Verification items for this drawing (mm, ordinates from the low corner). A direction names the side the tool comes from. Round coordinates to 2 decimals unless told otherwise and drop trailing zeros. Order: outer loops, then holes, each group sorted by start corner. A loop starts at its lowest first (then second) coordinate and runs counter-clockwise, first axis right, second up. Notation, with made-up numbers: (-3.75, -4) - (41.25, -4) arc R22 cw to (41.25, 20) - close; hole circle Ø8 at (-3.5, -32.75). An arc over 180 degrees is marked (long way). Answer as CSV lines item,"result". Start each with the question number.
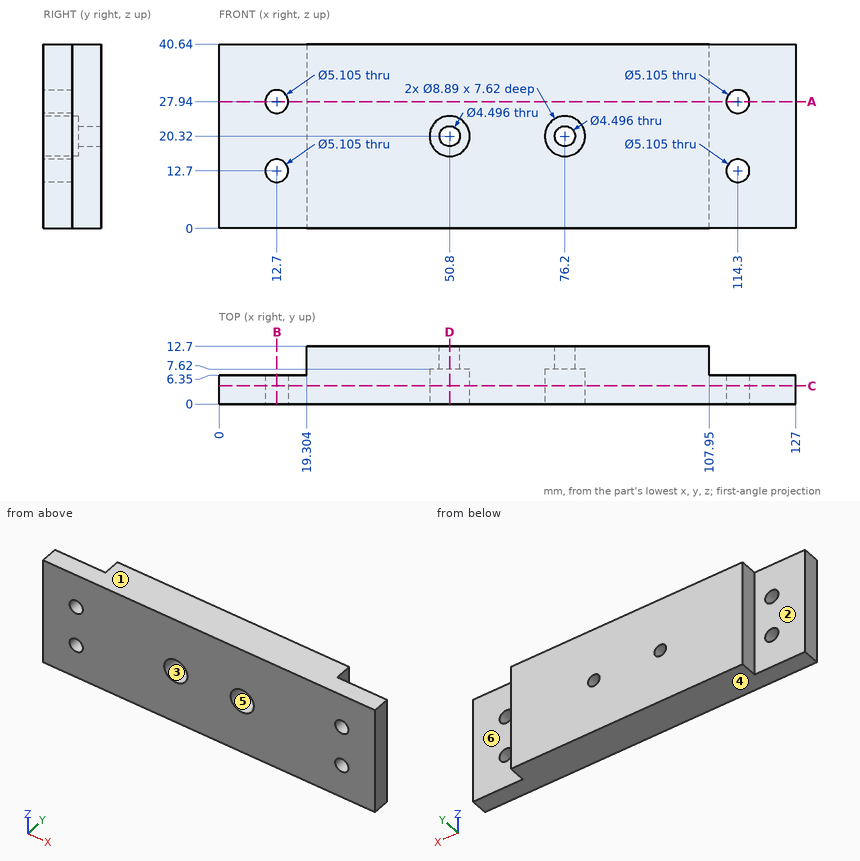
1. Section check B-B on x = 12.7. Record the boundary of the cut face in (y, z).
2. Section check D-D on x = 50.8. Record the boundary of the cut face in (y, z) (1 decimal).
3. Section check C-C on y = 4. Record the boundary of the cut face in (x, z) (1 decimal).
4. Go/stop test with flat-tipped pins: pin 1 Ø5 at (y, z) = (11, 20) entering from -X; pin 2 Ø8 at (x, z) = (114.3, 12.7) entering from +Y; pin 3 Ø2.5 at (x, z) = (50, 22.5) entering from -Y. Record where each tip stops, or that it passes through.
5. Thickness scan on probe 1 along X at (y, z) = (9.25, 20.32); probe 2 along Z at (x, y) = (50.8, 3.75) (1 decimal); probe 3 along X at (y, z) = (1.75, 27.94). Record the ranges inside material, lowest first.
6. Access from +Z, -Z, +X, -X, +Y, -Y to the whole of each face (thin tool, end or side, straight path). Record for the marked faces 1 and 2.
7. Section check A-A on z = 27.94. Record the boundary of the cut face in (x, y).
8. Draft check along Z on the marked faces 3, 4, 5 and 6. Enter one of: released by +Z, released by -Z, zero draft, split by the parting line, or undercut.
Numbers:
1,outline,"(0, 0) - (6.35, 0) - (6.35, 10.15) - (0, 10.15) - close; (0, 15.25) - (6.35, 15.25) - (6.35, 25.39) - (0, 25.39) - close; (0, 30.49) - (6.35, 30.49) - (6.35, 40.64) - (0, 40.64) - close"
2,outline,"(0, 0) - (12.7, 0) - (12.7, 18.1) - (7.6, 18.1) - (7.6, 15.9) - (0, 15.9) - close; (0, 24.8) - (7.6, 24.8) - (7.6, 22.6) - (12.7, 22.6) - (12.7, 40.6) - (0, 40.6) - close"
3,outline,"(0, 0) - (127, 0) - (127, 40.6) - (0, 40.6) - close; hole circle Ø5.1 at (12.7, 12.7); hole circle Ø5.1 at (12.7, 27.9); hole circle Ø8.9 at (50.8, 20.3); hole circle Ø8.9 at (76.2, 20.3); hole circle Ø5.1 at (114.3, 12.7); hole circle Ø5.1 at (114.3, 27.9)"
4,pin 1,"stops at x = 19.3"
4,pin 2,"stops at y = 6.35"
4,pin 3,"stops at y = 7.62"
5,probe 1,"x = 19.3 to 48.55, 53.05 to 73.95, 78.45 to 107.95"
5,probe 2,"z = 0 to 15.9, 24.8 to 40.6"
5,probe 3,"x = 0 to 10.15, 15.25 to 111.75, 116.85 to 127"
6,face 1,"+Z, +X, -X, +Y, -Y"
6,face 2,"+Z, -Z, -X, +Y"
7,outline,"(0, 0) - (10.15, 0) - (10.15, 6.35) - (0, 6.35) - close; (15.25, 0) - (111.75, 0) - (111.75, 6.35) - (107.95, 6.35) - (107.95, 12.7) - (19.3, 12.7) - (19.3, 6.35) - (15.25, 6.35) - close; (116.85, 0) - (127, 0) - (127, 6.35) - (116.85, 6.35) - close"
8,face 3,"undercut"
8,face 4,"released by -Z"
8,face 5,"undercut"
8,face 6,"zero draft"
